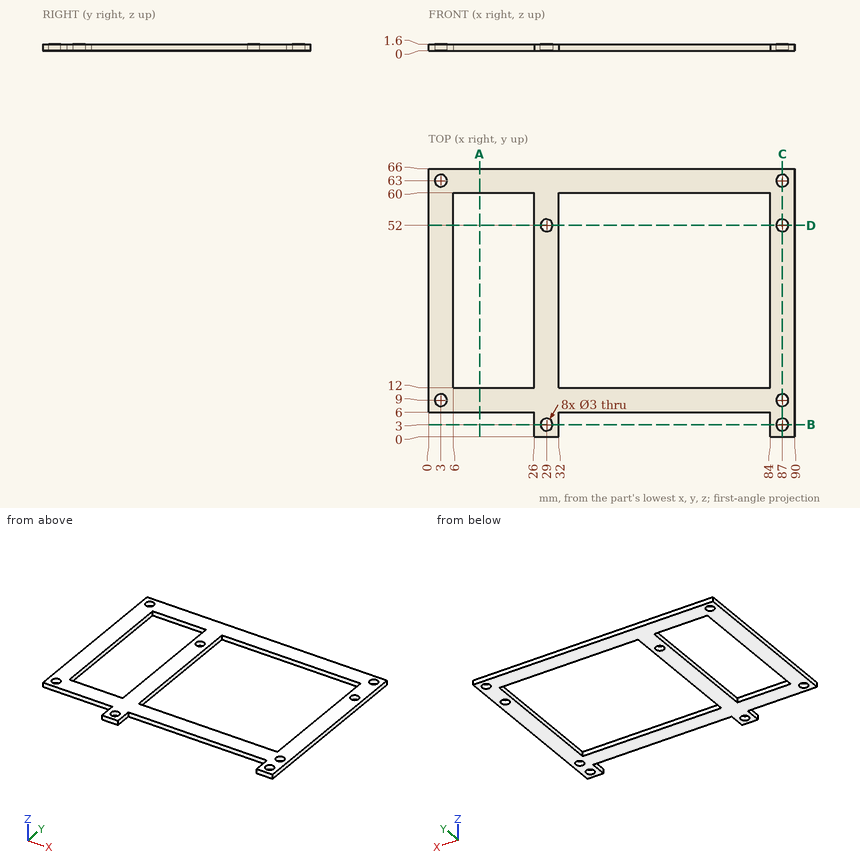
Verification items for this drawing (mm, ordinates from the low corner). Coordinates: 2 decimals unless noted, no trailing zeros. Loops run counter-clockwise (first coordinate to the right, second up) from the corner with the lowest first, then second, coordinate; pieces in that order, holes last. Notation, with made-up numbers: (9, 36.5) - (61, 36.5) arc R31 cw to (61, 66.5) - close; hole circle Ø11 at (47.25, 80). An arc over 180 degrees is marked (long way). One line per item, written item: value. Start each with the question number.
(1) Cross-section at C-C on x = 87. Enter the section's corners in (y, z), plus the area to 3 significant figures.
(2) Cross-section at B-B on y = 3. Enter the section's corners in (x, z).
(3) Depth check by flat-ended pin: P1, Ø1.5, axis at x = 34.5, y = 53.5, coming from the -Z side; P2, Ø0.5, axis at x = 15, z = 1, coming from the -Y side; P3, Ø0.8, axis at y = 3.5, z = 1, coming from the -X side. Enter the tip coordinate at first touch or a pass-through.
(4) Cross-section at D-D on y = 52. Enter the section's corners in (x, z).
(5) Cross-section at A-A on x = 12.5. Enter the section's corners in (y, z), plus the area to 3 significant figures.
(6) Material ranges on line 1 (Y direction, x = 87, z = 0.7); line 2 (X direction, y = 29, z = 0.5); line 3 (Y direction, x = 39, z = 1.25), recorded low to high. Write a range as [from, to].
Results below:
1. outline: (0, 0) - (1.5, 0) - (1.5, 1.6) - (0, 1.6) - close; (4.5, 0) - (7.5, 0) - (7.5, 1.6) - (4.5, 1.6) - close; (10.5, 0) - (50.5, 0) - (50.5, 1.6) - (10.5, 1.6) - close; (53.5, 0) - (61.5, 0) - (61.5, 1.6) - (53.5, 1.6) - close; (64.5, 0) - (66, 0) - (66, 1.6) - (64.5, 1.6) - close
1. area: 86.4 mm2
2. outline: (26, 0) - (27.5, 0) - (27.5, 1.6) - (26, 1.6) - close; (30.5, 0) - (32, 0) - (32, 1.6) - (30.5, 1.6) - close; (84, 0) - (85.5, 0) - (85.5, 1.6) - (84, 1.6) - close; (88.5, 0) - (90, 0) - (90, 1.6) - (88.5, 1.6) - close
3. P1: passes through
3. P2: stops at y = 6
3. P3: stops at x = 26
4. outline: (0, 0) - (6, 0) - (6, 1.6) - (0, 1.6) - close; (26, 0) - (27.5, 0) - (27.5, 1.6) - (26, 1.6) - close; (30.5, 0) - (32, 0) - (32, 1.6) - (30.5, 1.6) - close; (84, 0) - (85.5, 0) - (85.5, 1.6) - (84, 1.6) - close; (88.5, 0) - (90, 0) - (90, 1.6) - (88.5, 1.6) - close
5. outline: (6, 0) - (12, 0) - (12, 1.6) - (6, 1.6) - close; (60, 0) - (66, 0) - (66, 1.6) - (60, 1.6) - close
5. area: 19.2 mm2
6. line 1: y = [0, 1.5], [4.5, 7.5], [10.5, 50.5], [53.5, 61.5], [64.5, 66]
6. line 2: x = [0, 6], [26, 32], [84, 90]
6. line 3: y = [6, 12], [60, 66]
